Model file for the job. Use its own axes, mm. Give positions to 0.01 mm unless a question says otherwise; leave off trailing zeros. Order: outer loops, then holes, each group sorted by start corner. A loop starts at its lowest first (then second) coordinate and runs counter-clockwise, first axis right, second up. Notation, with made-up numbers: (84, -7) -> (90, -7) arc R36 ccw to (90, 31) -> close; hole circle Ø3 at (11.25, 59). An arc over 180 degrees is marked (long way). Use CSV: the item, a comma, the result in double quotes. Start each with the question number.
1. Cut at D-D on y = 0.75. List the corners of the cut face in (x, z).
2. Drop flat-ended pins along their axis: pin 1 (1.5 mm diameter, centred on x = 1, z = -3, fed in from +Y); pin 2 (1 mm diameter, centred on x = -1, y = 8, fed in from +Z); pin 3 (1 mm diameter, centred on x = -4, y = 2, fed in from -Z); pin 4 (1.5 mm diameter, centred on x = 4.5, y = 6.5, fed in from +Z). Give the stop position or say it passes through.
3. Wall check: line 1 (X direction, y = 4.5, z = 0); line 2 (X direction, y = 3.25, z = 3.5); line 3 (Z direction, x = 2.5, y = 6.25). Give the ranges that are in metal, low to high. Write a range as from..to.
4. Pull direction X, two halves, no side cores. Call faces 1 (the cylindrical face through (1.802, 4.944, 5.723)), 2 (the cylindrical face through (-3.905, 4.944, -0.867)): released by +X, released by -X, zero draft, split by the parting line, or undercut.
5. Cut at C-C on y = 8. List the corners of the cut face in (x, z).
```python
from build123d import *

# Parameters (mm, degrees)
SKETCH_1_R      = 6
SKETCH_1_R_2    = 4
EXTRUDE_1_DEPTH = 10
FILLET_1_R      = 1


with BuildPart() as part:
    # Эскиз1 → Бобышка-Вытянуть1 (new body)
    with BuildSketch(Plane(origin=(0, 0, 0), x_dir=(1, 0, 0), z_dir=(0, 1, 0))):
        with Locations(Location((0, 0, 0), (0, 0, 270))):
            Circle(SKETCH_1_R)
        with Locations(Location((0, 0, 0), (0, 0, 270))):
            Circle(SKETCH_1_R_2, mode=Mode.SUBTRACT)
    extrude(amount=EXTRUDE_1_DEPTH)

    # 圆角1
    fillet_1_edges = [part.edges().sort_by_distance(p)[0] for p in [
        (0, 0, -6),
        (0, 10, -6),
        (0, 0, -4),
        (0, 10, -4),
    ]]
    fillet(fillet_1_edges, radius=FILLET_1_R - 0.0001)  # a hair under: the kernel refuses the full size


solid = part.part
```
Verdict:
1,outline,"circle Ø11.94 at (0, 0); hole circle Ø8.06 at (0, 0)"
2,pin 1,"through"
2,pin 2,"z = 5.98"
2,pin 3,"z = -4.87"
2,pin 4,"z = 4.68"
3,line 1,"-6..-4, 4..6"
3,line 2,"-4.87..-1.94, 1.94..4.87"
3,line 3,"-5.45..-3.12, 3.12..5.45"
4,face 1,"split by the parting line"
4,face 2,"undercut"
5,outline,"circle Ø12 at (0, 0); hole circle Ø8 at (0, 0)"
